from build123d import *

# Parameters (mm, degrees)
SKETCH1_R           = 2.05
SKETCH1_R_2         = 1.5
BOSS_EXTRUDE1_DEPTH = 3


with BuildPart() as part:
    # Sketch1 → Boss-Extrude1 (new body)
    with BuildSketch(Plane.XY.offset(3)):
        with BuildLine():
            Line((-12, -26.830532015), (-12, -33))
            ThreePointArc((-12, -33), (-11.414213562, -34.414213562), (-10, -35))
            Line((-10, -35), (10, -35))
            ThreePointArc((10, -35), (11.414213562, -34.414213562), (12, -33))
            Line((12, -33), (12, -26.830532015))
            ThreePointArc((12, -26.830532015), (12.746170978, -22.15844916), (14.910447761, -17.951189322))
            ThreePointArc((14.910447761, -17.951189322), (0, 11.5), (-14.910447761, -17.951189322))
            ThreePointArc((-14.910447761, -17.951189322), (-12.746170978, -22.15844916), (-12, -26.830532015))
        make_face()
        with Locations(Location((8, -31, 0), (0, 0, 180))):
            Circle(SKETCH1_R, mode=Mode.SUBTRACT)
        with Locations(Location((-8, -31, 0), (0, 0, 180))):
            Circle(SKETCH1_R, mode=Mode.SUBTRACT)
        with Locations(Location((0, -31, 0), (0, 0, 180))):
            Circle(SKETCH1_R, mode=Mode.SUBTRACT)
        with Locations(Location((-7.75, 6.423393759, 0), (0, 0, 180))):
            Circle(SKETCH1_R_2, mode=Mode.SUBTRACT)
        with Locations(Location((7.75, 6.423393759, 0), (0, 0, 180))):
            Circle(SKETCH1_R_2, mode=Mode.SUBTRACT)
        with Locations(Location((15.5, -7, 0), (0, 0, 180))):
            Circle(SKETCH1_R_2, mode=Mode.SUBTRACT)
        with Locations(Location((7.75, -20.423393759, 0), (0, 0, 180))):
            Circle(SKETCH1_R_2, mode=Mode.SUBTRACT)
        with Locations(Location((-7.75, -20.423393759, 0), (0, 0, 180))):
            Circle(SKETCH1_R_2, mode=Mode.SUBTRACT)
        with Locations(Location((-15.5, -7, 0), (0, 0, 180))):
            Circle(SKETCH1_R_2, mode=Mode.SUBTRACT)
        with Locations(Location((-8.5, -7, 0), (0, 0, 180))):
            Circle(SKETCH1_R_2, mode=Mode.SUBTRACT)
        with Locations(Location((0, -23, 0), (0, 0, 180))):
            Circle(SKETCH1_R, mode=Mode.SUBTRACT)
        with Locations(Location((8.5, -7, 0), (0, 0, 180))):
            Circle(SKETCH1_R_2, mode=Mode.SUBTRACT)
        with BuildLine():
            ThreePointArc((3.23332646, -5.66), (0, -10.5), (-3.23332646, -5.66))
            ThreePointArc((-3.23332646, -5.66), (-3.216371052, -5.324717761), (-3.415288556, -5.054285714))
            ThreePointArc((-3.415288556, -5.054285714), (0, 6.1), (3.415288556, -5.054285714))
            ThreePointArc((3.415288556, -5.054285714), (3.216371052, -5.324717761), (3.23332646, -5.66))
        make_face(mode=Mode.SUBTRACT)
        with BuildLine():
            ThreePointArc((6.01040764, -13.01040764), (8.131727984, -13.01040764), (8.131727984, -15.131727984))
            ThreePointArc((8.131727984, -15.131727984), (0, -18.5), (-8.131727984, -15.131727984))
            ThreePointArc((-8.131727984, -15.131727984), (-8.131727984, -13.01040764), (-6.01040764, -13.01040764))
            ThreePointArc((-6.01040764, -13.01040764), (0, -15.5), (6.01040764, -13.01040764))
        make_face(mode=Mode.SUBTRACT)
    extrude(amount=-BOSS_EXTRUDE1_DEPTH)


solid = part.part
Model file for the job. Use its own axes, mm. A direction names the side the tool comes from. Coordinates: 2 decimals unless noted, no trailing zeros. Loops run counter-clockwise (first coordinate to the right, second up) from the corner with the lowest first, then second, coordinate; pieces in that order, holes last. Notation, with made-up numbers: (-39.5, 81) -> (-17.5, 81) arc R26 ccw to (-17.5, 101) -> close; hole circle Ø10 at (77, 76). An arc over 180 degrees is marked (long way). Use one line per item in the form item = value. Start each with the question number.
(1) Cut at C-C on z = 1.1. Give the number of separate pieces and of enclosed holes in the cut face, and give its area (3 significant figures).
(2) Probe probe 1 along X at (y, z) = (-7, 1.6); probe 2 along Y at (x, z) = (0, 1.9); probe 3 along X at (y, z) = (-31, 0.45). List the from-to ranges inside material, lowest first. Write a range as from..to.
(3) Flat gauge pin, fed straight in: pin 1 (1.5 mm diameter, centred on y = -10.5, z = 0.5, fed in from -X). Where does the tip first touch, or does it go through?
(4) Pull direction Y, two halves, no side cores. Call faces 1 (the cylindrical face through (9.7, -6.1, 1.5)), 2 (the cylindrical face through (-11.43, -34.4, 1.52)), 3 (the flat face through (12, -30, 2)): pulls with the +Y half, pulls with the -Y half, needs draft (parallel to the pull), parting line crosses it, or undercut.
(5) Tool access for faces 4 (the flat face through (0, -35, 2)), 5 (the cylindrical face through (-0.1, -15.5, 1.5)): list every direction of +Z, -Z, +X, -X, +Y, -Y with a clear straight run to the whole face (end or side of a thin tool).
(6) Cut at D-D on y = -9.5. Give the cut face in (x, z), and give its area (3 significant figures).
(7) Cut at A-A on y = -31. Give the cut face in (x, z).
(8) Cut at B-B on x = -15.5. Give the cut face in (y, z).
Values:
q1.separate_pieces = 1
q1.enclosed_holes = 14
q1.area = 1,030 mm2
q2.probe_1 = -18.5..-17, -14..-10, -7..-3.5, 3.5..7, 10..14, 17..18.5
q2.probe_2 = -35..-33.05, -28.95..-25.05, -20.95..-18.5, -15.5..-10.5, 6.1..11.5
q2.probe_3 = -12..-10.05, -5.95..-2.05, 2.05..5.95, 10.05..12
q3.pin_1 = -18.29
q4.face_1 = undercut
q4.face_2 = pulls with the -Y half
q4.face_3 = needs draft
q5.face_4 = +Z, -Z, +X, -X, -Y
q5.face_5 = +Z, -Z
q6.outline = (-18.33, 0) -> (-2.45, 0) -> (-2.45, 3) -> (-18.33, 3) -> close; (2.45, 0) -> (18.33, 0) -> (18.33, 3) -> (2.45, 3) -> close
q6.area = 95.3 mm2
q7.outline = (-12, 0) -> (-10.05, 0) -> (-10.05, 3) -> (-12, 3) -> close; (-5.95, 0) -> (-2.05, 0) -> (-2.05, 3) -> (-5.95, 3) -> close; (2.05, 0) -> (5.95, 0) -> (5.95, 3) -> (2.05, 3) -> close; (10.05, 0) -> (12, 0) -> (12, 3) -> (10.05, 3) -> close
q8.outline = (-17.1, 0) -> (-8.5, 0) -> (-8.5, 3) -> (-17.1, 3) -> close; (-5.5, 0) -> (3.1, 0) -> (3.1, 3) -> (-5.5, 3) -> close
